For this review, take the finished solid that the model builds, in its own axes (mm). Face numbers are marked on the shaded views. A direction names the side the tool comes from. Give positions to 0.01 mm unless a question says otherwise; leave off trailing zeros. Order: outer loops, then holes, each group sorted by start corner. A loop starts at its lowest first (then second) coordinate and runs counter-clockwise, first axis right, second up. Notation, with made-up numbers: (71.5, -22.5) - (87.5, -22.5) arc R16 ccw to (87.5, -18.5) - close; hole circle Ø1 at (22.5, 88.5). An arc over 180 degrees is marked (long way). One line per item, written item: value.
```python
from build123d import *

# Parameters (mm, degrees)
BOSS_EXTRUDE1_DEPTH            = 6.35
F_3_16_0_1875_DIAMETER_HOLE1_D = 4.7625
F_21_0_159_DIAMETER_HOLE1_D    = 4.0386
SKETCH4_W                      = 15.875
SKETCH4_H                      = 12.7
CUT_EXTRUDE1_DEPTH             = 3.175


with BuildPart() as part:
    # Sketch1 → Boss-Extrude1 (new body)
    with BuildSketch(Plane(origin=(0, 0, 0), x_dir=(1, 0, 0), z_dir=(0, 1, 0))):
        with BuildLine():
            Line((-39.6875, 6.35), (39.6875, 6.35))
            ThreePointArc((39.6875, 6.35), (46.0375, 0), (39.6875, -6.35))
            Line((39.6875, -6.35), (-39.6875, -6.35))
            ThreePointArc((-39.6875, -6.35), (-46.0375, 0), (-39.6875, 6.35))
        make_face()
    extrude(amount=BOSS_EXTRUDE1_DEPTH)

    # 3/16 (0.1875) Diameter Hole1 (through all)
    with Locations(Plane(origin=(0, 6.35, 0), x_dir=(1, 0, 0), z_dir=(0, 1, 0))):
        with Locations((-39.6875, 0)):
            Hole(F_3_16_0_1875_DIAMETER_HOLE1_D / 2)

    # #21 (0.159) Diameter Hole1 (through all)
    with Locations(Plane(origin=(0, 6.35, 0), x_dir=(1, 0, 0), z_dir=(0, 1, 0))):
        with Locations((39.6875, 0)):
            Hole(F_21_0_159_DIAMETER_HOLE1_D / 2)

    # Sketch4 → Cut-Extrude1 (cut)
    with BuildSketch(Plane(origin=(0, 6.35, 0), x_dir=(1, 0, 0), z_dir=(0, 1, 0))):
        with Locations((39.6875, 0)):
            Rectangle(SKETCH4_W, SKETCH4_H)
    extrude(amount=-CUT_EXTRUDE1_DEPTH, mode=Mode.SUBTRACT)


solid = part.part
```
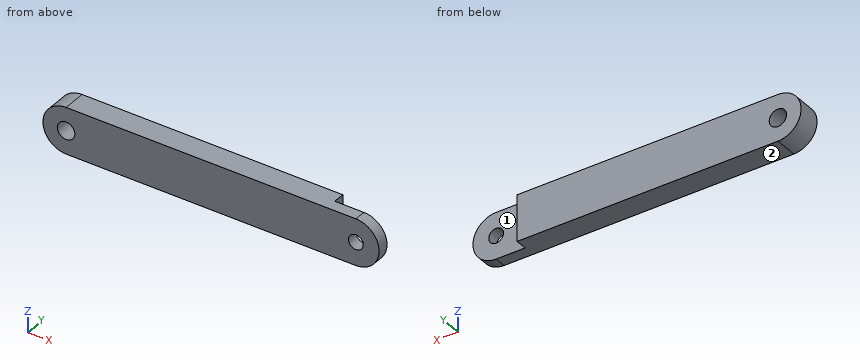
(1) Machinability: for the marked faces 1 and 2, which of the approach directions +Z, -Z, +X, -X, +Y, -Y give a long, thin tool a straight path to every point of the face, cutting with its end or side? Answer none if there is none.
Answers below:
face 1: +Z, -Z, +X, +Y
face 2: -Z, +X, -X, +Y, -Y
(2) For P1, Ø1.5, axis at y = 3, z = 4, coming from the +X side; P2, Ø5.5, axis at x = 39.69, z = 0, coming from the +Y side (3 decimals); P3, Ø3.5, axis at y = 5, z = -1.5, coming from the +X side, all flat-tipped, find the tip position at first contact; note any pin that passes through.
Answers below:
P1: stops at x = 45.14
P2: stops at y = 3.175
P3: stops at x = 31.75
(3) Take a section at A-A (z = 0). Give the number of separate pieces and of enclosed holes in the cut face, then the cut area to 3 significant figures.
Answers below:
separate pieces: 3
enclosed holes: 0
area: 496 mm^2
(4) Wall thickness on line 1 (X direction, y = 2, z = 0.25); line 2 (X direction, y = 0.5, z = 1); line 3 (Y direction, x = 34, z = 3.75) (3 decimals): over which ranges is each line inside the solid? List them lowest first. Write a range as from..to.
Answers below:
line 1: x = -46.03..-42.06, -37.32..37.68, 41.69..46.03
line 2: x = -45.96..-41.85, -37.53..37.93, 41.44..45.96
line 3: y = 0..3.175
(5) Take a section at C-C (x = 34). Write out the cut boundary in (y, z) (3 decimals), then the cut area to 3 significant figures.
Answers below:
outline: (0, -6.35) - (3.175, -6.35) - (3.175, 6.35) - (0, 6.35) - close
area: 40.3 mm^2
(6) Take a section at B-B (y = 5.5). Write out the cut boundary in (x, z), then the cut area to 3 significant figures.
Answers below:
outline: (-39.69, -6.35) - (31.75, -6.35) - (31.75, 6.35) - (-39.69, 6.35) arc R6.35 ccw to start; hole circle Ø4.76 at (-39.69, 0)
area: 953 mm^2
